Source: CAD feature listing. Evaluate the final solid. Frame: model axes, mm. Face numbers are marked on the shaded views. Give positions to 0.01 mm unless a question says otherwise; leave off trailing zeros. Loops run counter-clockwise (first coordinate to the right, second up) from the corner with the lowest first, then second, coordinate; pieces in that order, holes last. Notation, with made-up numbers: (40, 88.25) -> (69, 88.25) arc R19 ccw to (69, 117.25) -> close; hole circle Ø6 at (-6.5, -8). An arc over 180 degrees is marked (long way). Put each result on its own line as item: value.
Autodesk Inventor part; units mm, degrees
ref_plane "YZ Plane" through (0, 0, 0) normal (1, 0, 0) x (0, 1, 0)
ref_plane "XZ Plane" through (0, 0, 0) normal (0, 1, 0) x (-1, 0, 0)
ref_plane "XY Plane" through (0, 0, 0) normal (0, 0, 1) x (1, 0, 0)
sketch "Sketch1" plane through (0, 0, 0) normal (0, 0, 1) x (1, 0, 0)
  line L0 (-30, 9.2) -> (30, 9.2)
  line L1 (30, 9.2) -> (30, 3.2)
  line L2 (30, 3.2) -> (25.875, 3.2)
  line L3 (25, 2.325) -> (25, -10.2)
  line L4 (24.5, -10.7) -> (20.5, -10.7)
  line L5 (20, -10.2) -> (20, -10.075)
  line L6 (19.125, -9.2) -> (4.875, -9.2)
  line L7 (4, -10.075) -> (4, -10.2)
  line L8 (3.5, -10.7) -> (-3.5, -10.7)
  line L9 (-4, -10.2) -> (-4, -10.075)
  line L10 (-4.875, -9.2) -> (-19.125, -9.2)
  line L11 (-20, -10.075) -> (-20, -10.2)
  line L12 (-20.5, -10.7) -> (-24.5, -10.7)
  line L13 (-25, -10.2) -> (-25, 2.325)
  line L14 (-25.875, 3.2) -> (-30, 3.2)
  line L15 (-30, 3.2) -> (-30, 9.2)
  line L16 (0, 7.251) -> (0, -4.9434) construction
  line L17 (-9.4671, 0) -> (8.147, 0) construction
  arc A0 (-25, 2.325) -> (-25.875, 3.2) centre (-25.875, 2.325) ccw
  arc A1 (25.875, 3.2) -> (25, 2.325) centre (25.875, 2.325) ccw
  line L18 (-25, -10.2) -> (-24.5, -10.7)
  line L19 (-20, -10.2) -> (-20.5, -10.7)
  line L20 (-4, -10.2) -> (-3.5, -10.7)
  line L21 (3.5, -10.7) -> (4, -10.2)
  line L22 (20, -10.2) -> (20.5, -10.7)
  line L23 (25, -10.2) -> (24.5, -10.7)
  arc A2 (-19.125, -9.2) -> (-20, -10.075) centre (-19.125, -10.075) ccw
  arc A3 (-4, -10.075) -> (-4.875, -9.2) centre (-4.875, -10.075) ccw
  arc A4 (4.875, -9.2) -> (4, -10.075) centre (4.875, -10.075) ccw
  arc A5 (20, -10.075) -> (19.125, -9.2) centre (19.125, -10.075) ccw
  point P0 (0, 0)
  dimension "d0" = 8
  dimension "d1" = 1.5
  dimension "d2" = 5
  dimension "d3" = 20
  dimension "d4" = 18.4
  dimension "d6" = 6
  dimension "d7" = 5
  dimension "d19" = 45
  dimension "d20" = 0.5
  dimension "d23" = 1.75
extrude "Extrusion1" add sketch "Sketch1" along normal blind 1.6
sketch "Sketch2" plane through (0, 0, 1.6) normal (0, 0, 1) x (1, 0, 0)
  line L0 (-30, 9.2) -> (30, 9.2)
  point P0 (0, 0)
  point P1 (0, -1.3)
  point P2 (-16, -1.3)
  point P3 (16, -1.3)
  dimension "d10" = 16
  dimension "d11" = 16
  dimension "d21" = 10.5
hole "Hole1" at (0, -1.3, 1.6) at (-16, -1.3, 1.6) at (16, -1.3, 1.6) direction (0, 0, -1) diameter 1 end through all
properties part number "AK-C-C39-Pinhole-Board"
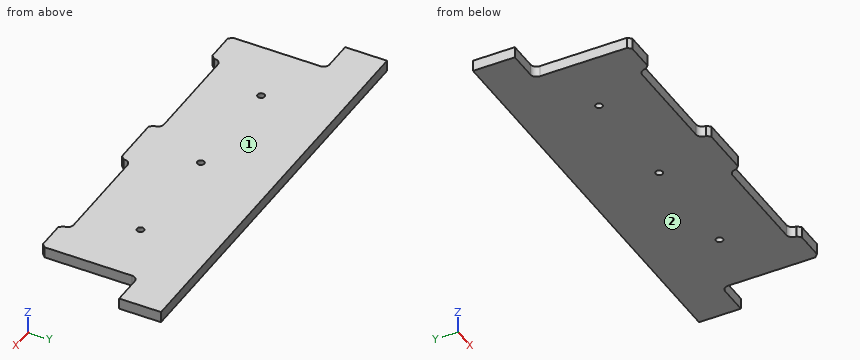
(1) Section B-B on x = 9. Return loops of the section in (y, z).
Calculated:
outline: (-9.2, 0) -> (9.2, 0) -> (9.2, 1.6) -> (-9.2, 1.6) -> close
(2) Section A-A on y = -7.25. Return loops of the section in (x, z), then the cut area to 3 significant figures.
Calculated:
outline: (-25, 0) -> (25, 0) -> (25, 1.6) -> (-25, 1.6) -> close
area: 80.0 mm²
(3) Draft query along Z for the marked faces 1 and 2. Return one class per face: released by +Z, released by -Z, zero draft, split by the parting line, or undercut.
Calculated:
face 1: released by +Z
face 2: released by -Z
(4) Line query: probe 1 along X at (y, z) = (-1.3, 1); probe 2 along Y at (x, z) = (-16, 0.7); probe 3 along X at (y, z) = (1.5, 0.4). Output: solid intervals per line, ascending. Write a range as from..to.
Calculated:
probe 1: x = -25..-16.5, -15.5..-0.5, 0.5..15.5, 16.5..25
probe 2: y = -9.2..-1.8, -0.8..9.2
probe 3: x = -25..25
